Part print with two shaded views. Sizes in mm from the minimum x, y, z corner. Round coordinates to 2 decimals unless told otherwise and drop trailing zeros. Order: outer loops, then holes, each group sorted by start corner. A loop starts at its lowest first (then second) coordinate and runs counter-clockwise, first axis right, second up. Notation, with made-up numbers: M -16,61 L -8,61 A15 ccw -8,71 Z; hole C 81.25,-21.75 d1. An arc over 180 degrees is marked long. Return JSON: item names as keys, results as strings. Group by question number.
Item 1: Slice it at C-C on x = 21. Write the cut outline in (y, z), then the cut area to 3 significant figures.
Item 2: Pin check, flat tips, straight feed: pin 1 Ø6 at (x, y) = (92.5, 72.5) entering from -Z; pin 2 Ø10.5 at (x, y) = (97.12, 97.12) entering from +Z; pin 3 Ø12 at (y, z) = (66.5, 4.5) entering from -X; pin 4 Ø12 at (x, z) = (77.5, 24.5) entering from -Y. Stop position of each tip, or through.
Item 3: Probe line 1 along Y through (x, z) = (60, 32); line 2 along X through (y, z) = (59.5, 20.5); line 3 along Z through (x, y) = (15.5, 44). List the from-to ranges inside material, lowest first.
Item 4: Slice it at A-A on y = 60. Write the cut outline in (x, z).
Item 5: Slice it at D-D on z = 3.5. Write the cut outline in (x, y).
Item 6: Pull direction X, two halves, no side cores. Call the marked faces 1, 2 and 3: pulls with the +X half, pulls with the -X half, needs draft (parallel to the pull), parting line crosses it, or undercut.
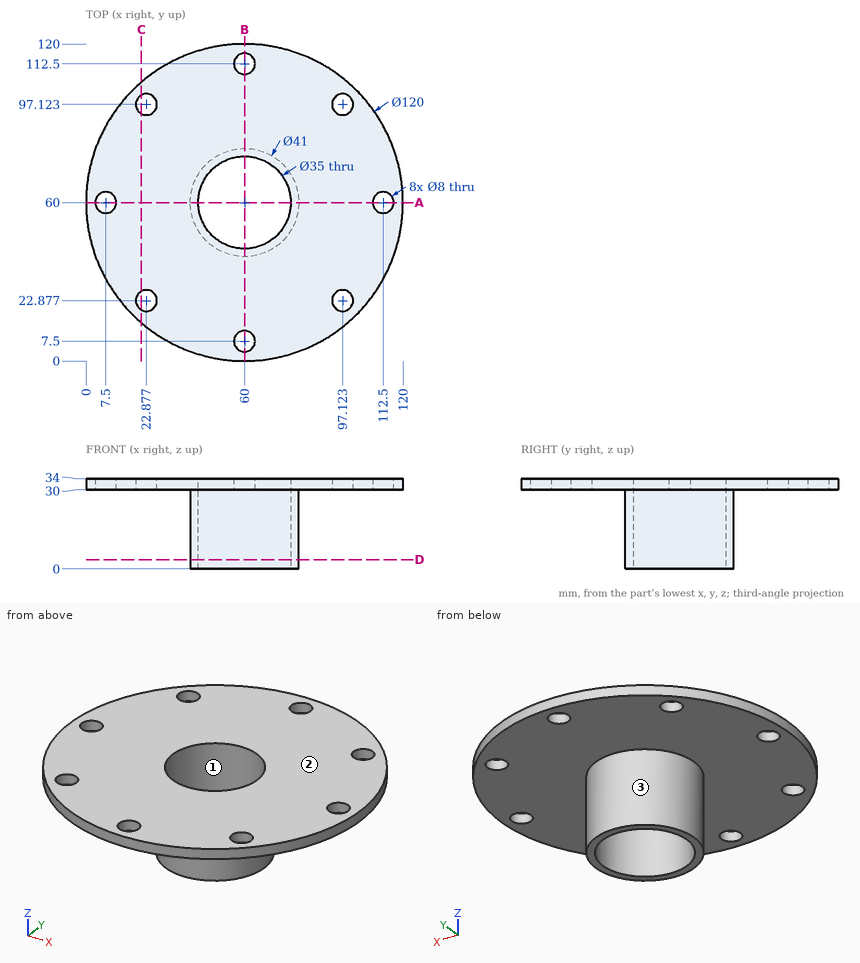
Output values:
{
 "1": {"outline": "M 14.4,30 L 19.34,30 L 19.34,34 L 14.4,34 Z; M 26.41,30 L 93.59,30 L 93.59,34 L 26.41,34 Z; M 100.66,30 L 105.6,30 L 105.6,34 L 100.66,34 Z", "area": "308 mm²"},
 "2": {"pin 1": "z = 30", "pin 2": "z = 34", "pin 3": "x = 39.51", "pin 4": "y = 1.93"},
 "3": {"line 1": "0 to 3.5, 11.5 to 42.5, 77.5 to 108.5, 116.5 to 120", "line 2": "39.51 to 42.51, 77.49 to 80.49", "line 3": "30 to 34"},
 "4": {"outline": "M 0,30 L 3.5,30 L 3.5,34 L 0,34 Z; M 11.5,30 L 39.5,30 L 39.5,0 L 42.5,0 L 42.5,34 L 11.5,34 Z; M 77.5,0 L 80.5,0 L 80.5,30 L 108.5,30 L 108.5,34 L 77.5,34 Z; M 116.5,30 L 120,30 L 120,34 L 116.5,34 Z"},
 "5": {"outline": "C 60,60 d41; hole C 60,60 d35"},
 "6": {"face 1": "undercut", "face 2": "needs draft", "face 3": "parting line crosses it"}
}
